from build123d import *

# Parameters (mm, degrees)
SKETCH1_W           = 20.5
SKETCH1_H           = 40.64
BOSS_EXTRUDE1_DEPTH = 39.5
CUT_EXTRUDE1_DEPTH  = 21.5
SKETCH3_W           = 55.64
SKETCH3_H           = 2.5
BOSS_EXTRUDE2_DEPTH = 20.5
SKETCH4_R           = 2.125
CUT_EXTRUDE2_DEPTH  = 33
SKETCH5_W           = 2.5
SKETCH5_H           = 1.601534114
CUT_EXTRUDE3_DEPTH  = 33
BOSS_EXTRUDE3_DEPTH = 1
SKETCH7_R           = 6.5
BOSS_EXTRUDE4_DEPTH = 1.5
SKETCH8_R           = 2.9
BOSS_EXTRUDE5_DEPTH = 1.25
SKETCH9_R           = 4.445
BOSS_EXTRUDE6_DEPTH = 3
SKETCH10_R          = 10.4
BOSS_EXTRUDE7_DEPTH = 2
SKETCH11_R          = 1.25
CUT_EXTRUDE4_DEPTH  = 7.75
SKETCH12_R          = 3.45
SKETCH12_R_2        = 2.85
BOSS_EXTRUDE8_DEPTH = 0.7
SKETCH13_R          = 0.4
CUT_EXTRUDE5_DEPTH  = 2
FILLET1_R           = 1.5
FILLET2_R           = 0.5
CUT_EXTRUDE6_START  = -7.75
CUT_EXTRUDE6_DEPTH  = 0.5
CUT_EXTRUDE7_DEPTH  = 0.5
SKETCH16_W          = 50.439593456
SKETCH16_H          = 8.25
CUT_EXTRUDE8_DEPTH  = 21.65
SKETCH17_R          = 8.5
BOSS_EXTRUDE9_DEPTH = 4


with BuildPart() as part:
    # Sketch1 → Boss-Extrude1 (new body)
    with BuildSketch(Plane(origin=(0, 0, 0), x_dir=(1, 0, 0), z_dir=(0, 1, 0))):
        with Locations((0, 20.32)):
            Rectangle(SKETCH1_W, SKETCH1_H)
    extrude(amount=BOSS_EXTRUDE1_DEPTH)

    # Sketch2 → Cut-Extrude1 (cut, through all)
    with BuildSketch(Plane(origin=(10.25, 0, 0), x_dir=(0, 0, -1), z_dir=(1, 0, 0))):
        Polygon((0, 39.5), (0, 36.35), (8, 39.5), align=None)
    extrude(amount=-CUT_EXTRUDE1_DEPTH, mode=Mode.SUBTRACT)

    # Sketch3 → Boss-Extrude2 (add)
    with BuildSketch(Plane(origin=(10.25, 0, 0), x_dir=(0, 0, -1), z_dir=(1, 0, 0))):
        with Locations((20.32, 30.75)):
            Rectangle(SKETCH3_W, SKETCH3_H)
    extrude(amount=-BOSS_EXTRUDE2_DEPTH)

    # Sketch4 → Cut-Extrude2 (cut, through all)
    with BuildSketch(Plane(origin=(0, 32, 0), x_dir=(1, 0, 0), z_dir=(0, 1, 0))):
        with Locations((-5, -4.18)):
            Circle(SKETCH4_R)
        with Locations((5, -4.18)):
            Circle(SKETCH4_R)
        with Locations((5, 44.82)):
            Circle(SKETCH4_R)
        with Locations((-5, 44.82)):
            Circle(SKETCH4_R)
    extrude(amount=-CUT_EXTRUDE2_DEPTH, mode=Mode.SUBTRACT)

    # Sketch5 → Cut-Extrude3 (cut, through all)
    with BuildSketch(Plane(origin=(0, 32, 0), x_dir=(1, 0, 0), z_dir=(0, 1, 0))):
        with Locations((5, -6.699232943)):
            Rectangle(SKETCH5_W, SKETCH5_H)
        with Locations((-5, -6.699232943)):
            Rectangle(SKETCH5_W, SKETCH5_H)
        with Locations((-5, 47.339232943)):
            Rectangle(SKETCH5_W, SKETCH5_H)
        with Locations((5, 47.339232943)):
            Rectangle(SKETCH5_W, SKETCH5_H)
    extrude(amount=-CUT_EXTRUDE3_DEPTH, mode=Mode.SUBTRACT)

    # Sketch6 → Boss-Extrude3 (add, symmetric)
    with BuildSketch(Plane(origin=(0, 0, 0), x_dir=(0, 0, -1), z_dir=(1, 0, 0))):
        Polygon((0, 32), (-5, 32), (0, 34.5), align=None)
        Polygon((40.64, 32), (45.64, 32), (40.64, 34.5), align=None)
    extrude(amount=BOSS_EXTRUDE3_DEPTH, both=True)

    # Sketch7 → Boss-Extrude4 (add)
    with BuildSketch(Plane(origin=(0, 39.5, 0), x_dir=(1, 0, 0), z_dir=(0, 1, 0))):
        with Locations((0, 30.14)):
            Circle(SKETCH7_R)
    extrude(amount=BOSS_EXTRUDE4_DEPTH)

    # Sketch8 → Boss-Extrude5 (add)
    with BuildSketch(Plane(origin=(0, 41, 0), x_dir=(1, 0, 0), z_dir=(0, 1, 0))):
        with Locations((0, 30.14)):
            Circle(SKETCH8_R)
    extrude(amount=BOSS_EXTRUDE5_DEPTH)

    # Sketch9 → Boss-Extrude6 (add)
    with BuildSketch(Plane(origin=(0, 42.25, 0), x_dir=(1, 0, 0), z_dir=(0, 1, 0))):
        with Locations((0, 30.14)):
            Circle(SKETCH9_R)
    extrude(amount=BOSS_EXTRUDE6_DEPTH)

    # Sketch10 → Boss-Extrude7 (add)
    with BuildSketch(Plane(origin=(0, 45.25, 0), x_dir=(1, 0, 0), z_dir=(0, 1, 0))):
        with Locations((0, 30.14)):
            Circle(SKETCH10_R)
    extrude(amount=BOSS_EXTRUDE7_DEPTH)

    # Sketch11 → Cut-Extrude4 (cut)
    with BuildSketch(Plane(origin=(0, 47.25, 0), x_dir=(1, 0, 0), z_dir=(0, 1, 0))):
        with Locations((0, 30.14)):
            Circle(SKETCH11_R)
    extrude(amount=-CUT_EXTRUDE4_DEPTH, mode=Mode.SUBTRACT)

    # Sketch12 → Boss-Extrude8 (add)
    with BuildSketch(Plane(origin=(0, 47.25, 0), x_dir=(1, 0, 0), z_dir=(0, 1, 0))):
        with Locations((0, 30.14)):
            Circle(SKETCH12_R)
        with Locations((0, 30.14)):
            Circle(SKETCH12_R_2, mode=Mode.SUBTRACT)
    extrude(amount=BOSS_EXTRUDE8_DEPTH)

    # Sketch13 → Cut-Extrude5 (cut)
    with BuildSketch(Plane(origin=(0, 47.25, 0), x_dir=(1, 0, 0), z_dir=(0, 1, 0))):
        with Locations((0, 37.265)):
            Circle(SKETCH13_R)
        with Locations((3.5, 37.265)):
            Circle(SKETCH13_R)
        with Locations((-3.5, 37.265)):
            Circle(SKETCH13_R)
        with Locations((7.125, 26.64)):
            Circle(SKETCH13_R)
        with Locations((7.125, 30.14)):
            Circle(SKETCH13_R)
        with Locations((7.125, 33.64)):
            Circle(SKETCH13_R)
        with Locations((-3.5, 23.015)):
            Circle(SKETCH13_R)
        with Locations((0, 23.015)):
            Circle(SKETCH13_R)
        with Locations((3.5, 23.015)):
            Circle(SKETCH13_R)
        with Locations((-7.125, 33.64)):
            Circle(SKETCH13_R)
        with Locations((-7.125, 30.14)):
            Circle(SKETCH13_R)
        with Locations((-7.125, 26.64)):
            Circle(SKETCH13_R)
    extrude(amount=-CUT_EXTRUDE5_DEPTH, mode=Mode.SUBTRACT)

    # Fillet1
    fillet1_edges = [part.edges().sort_by_distance(p)[0] for p in [
        (10.25, 34.175, 0),
        (-10.25, 34.175, 0),
        (-10.25, 14.75, -40.64),
        (10.25, 14.75, -40.64),
        (10.25, 14.75, 0),
        (-10.25, 14.75, 0),
        (-10.25, 35.75, -40.64),
        (10.25, 35.75, -40.64),
    ]]
    fillet(fillet1_edges, radius=FILLET1_R)

    # Fillet2
    fillet2_edges = [part.edges().sort_by_distance(p)[0] for p in [
        (-3.75, 30.75, -48.14),
        (-6.25, 30.75, -48.14),
        (3.75, 30.75, -48.14),
        (6.25, 30.75, -48.14),
        (10.25, 30.75, 7.5),
        (-10.25, 30.75, 7.5),
        (-10.25, 30.75, -48.14),
        (-3.75, 30.75, 7.5),
        (-6.25, 30.75, 7.5),
        (3.75, 30.75, 7.5),
        (6.25, 30.75, 7.5),
    ]]
    fillet(fillet2_edges, radius=FILLET2_R)

    # Sketch14 → Cut-Extrude6 (cut)
    with BuildSketch(Plane.XZ.offset(CUT_EXTRUDE6_START)):
        with BuildLine():
            Line((-8.75, -40.64), (8.75, -40.64))
            ThreePointArc((8.75, -40.64), (9.810660172, -40.200660172), (10.25, -39.14))
            Line((10.25, -39.14), (10.25, -1.5))
            ThreePointArc((10.25, -1.5), (9.810660172, -0.439339828), (8.75, 0))
            Line((8.75, 0), (-8.75, 0))
            ThreePointArc((-8.75, 0), (-9.810660172, -0.439339828), (-10.25, -1.5))
            Line((-10.25, -1.5), (-10.25, -39.14))
            ThreePointArc((-10.25, -39.14), (-9.810660172, -40.200660172), (-8.75, -40.64))
        make_face()
        with BuildLine():
            Line((8.75, -0.25), (-8.75, -0.25))
            ThreePointArc((-8.75, -0.25), (-9.633883476, -0.616116524), (-10, -1.5))
            Line((-10, -1.5), (-10, -39.14))
            ThreePointArc((-10, -39.14), (-9.633883476, -40.023883476), (-8.75, -40.39))
            Line((-8.75, -40.39), (8.75, -40.39))
            ThreePointArc((8.75, -40.39), (9.633883476, -40.023883476), (10, -39.14))
            Line((10, -39.14), (10, -1.5))
            ThreePointArc((10, -1.5), (9.633883476, -0.616116524), (8.75, -0.25))
        make_face(mode=Mode.SUBTRACT)
    extrude(amount=-CUT_EXTRUDE6_DEPTH, mode=Mode.SUBTRACT)

    # Sketch15 → Cut-Extrude7 (cut)
    with BuildSketch(Plane.XZ.offset(-29.5)):
        with BuildLine():
            Line((-8.75, -40.64), (8.75, -40.64))
            ThreePointArc((8.75, -40.64), (9.810660172, -40.200660172), (10.25, -39.14))
            Line((10.25, -39.14), (10.25, -1.5))
            ThreePointArc((10.25, -1.5), (9.810660172, -0.439339828), (8.75, 0))
            Line((8.75, 0), (-8.75, 0))
            ThreePointArc((-8.75, 0), (-9.810660172, -0.439339828), (-10.25, -1.5))
            Line((-10.25, -1.5), (-10.25, -39.14))
            ThreePointArc((-10.25, -39.14), (-9.810660172, -40.200660172), (-8.75, -40.64))
        make_face()
        with BuildLine():
            Line((10, -39.14), (10, -1.5))
            ThreePointArc((10, -1.5), (9.633883476, -0.616116524), (8.75, -0.25))
            Line((8.75, -0.25), (-8.75, -0.25))
            ThreePointArc((-8.75, -0.25), (-9.633883476, -0.616116524), (-10, -1.5))
            Line((-10, -1.5), (-10, -39.14))
            ThreePointArc((-10, -39.14), (-9.633883476, -40.023883476), (-8.75, -40.39))
            Line((-8.75, -40.39), (8.75, -40.39))
            ThreePointArc((8.75, -40.39), (9.633883476, -40.023883476), (10, -39.14))
        make_face(mode=Mode.SUBTRACT)
    extrude(amount=CUT_EXTRUDE7_DEPTH, mode=Mode.SUBTRACT)

    # Sketch16 → Cut-Extrude8 (cut, through all)
    with BuildSketch(Plane(origin=(10.25, 0, 0), x_dir=(0, 0, -1), z_dir=(1, 0, 0))):
        with Locations((25.219796728, 4.125)):
            Rectangle(SKETCH16_W, SKETCH16_H)
    extrude(amount=-CUT_EXTRUDE8_DEPTH, mode=Mode.SUBTRACT)

    # Sketch17 → Boss-Extrude9 (add)
    with BuildSketch(Plane.XZ.offset(-8.25)):
        with Locations((0, -10.5)):
            Circle(SKETCH17_R)
    extrude(amount=BOSS_EXTRUDE9_DEPTH)


solid = part.part
Design review of the part built by this model. Coordinates are the model's own, in mm. A direction names the side the tool comes from. Coordinates: 2 decimals unless noted, no trailing zeros. Order: outer loops, then holes, each group sorted by start corner. A loop starts at its lowest first (then second) coordinate and runs counter-clockwise, first axis right, second up.
Item 1: For pin 1 Ø10 at (x, y) = (2.5, 20) entering from -Z; pin 2 Ø10 at (y, z) = (31, -24.5) entering from -X; pin 3 Ø1.2 at (y, z) = (31, 6) entering from +X; pin 4 Ø4 at (x, z) = (-5, 4.18) entering from -Y, all flat-tipped, find the tip position at first contact; note any pin that passes through.
Item 2: For faces 1 (the flat face through (0, 42.25, -27)), 2 (the flat face through (-1, 33, 1)), 3 (the cylindrical face through (9.8, 35.8, -40.21)), 4 (the flat face through (0, 39.5, -30)), list the 3-axis set-ups (+Z, -Z, +X, -X, +Y, -Y) from which the entire face can be reached by the end or side of a thin tool; tool diameter is ignored.
Item 3: Take a section at C-C, the plane z = -21. Write out the cut boundary in (x, y), then the cut area to 3 significant figures.
Item 4: Take a section at B-B, the plane y = 21. Write out the cut boundary in (x, z), then the cut area to 3 significant figures.
Item 5: Take a section at D-D, the plane y = 43.5. Write out the cut boundary in (x, z) (3 decimals).
Item 6: The part is to be moulded in two halves that separate along Z. For faces 5 (the flat face through (0, 36, -40.64)), 6 (the flat face through (0.14, 37.9, -3.94)), 7 (the cylindrical face through (-0.62, 47.6, -27.36)), say which applies: pulls with the +Z half, pulls with the -Z half, needs draft (parallel to the pull), parting line crosses it, or undercut.
Item 7: For line 1 (Y direction, x = 6, z = -22); line 2 (Z direction, x = -3.5, y = 46.3) (3 decimals); line 3 (X direction, y = 46, z = -30), list the stretches that pass through material, from the lowest coordinate up.
Item 8: Take a section at A-A, the plane z = -44.82. Write out the cut boundary in (x, y) (3 decimals), then the cut area to 3 significant figures.
The answers:
1. pin 1: stops at z = -40.64
1. pin 2: stops at x = -10.25
1. pin 3: stops at x = 10.25
1. pin 4: passes through
2. face 1: none
2. face 2: +Z, -X, +Y
2. face 3: -Z, +X, +Y
2. face 4: +Y
3. outline: (-10.25, 8.25) - (10.25, 8.25) - (10.25, 29) - (10, 29) - (10, 29.5) - (10.25, 29.5) - (10.25, 39.5) - (-10.25, 39.5) - (-10.25, 29.5) - (-10, 29.5) - (-10, 29) - (-10.25, 29) - close; (-4.96, 45.25) - (4.96, 45.25) - (4.96, 47.25) - (-4.96, 47.25) - close
3. area: 660 mm2
4. outline: (-10.25, -39.14) arc R1.5 ccw to (-8.75, -40.64) - (8.75, -40.64) arc R1.5 ccw to (10.25, -39.14) - (10.25, -1.5) arc R1.5 ccw to (8.75, 0) - (-8.75, 0) arc R1.5 ccw to (-10.25, -1.5) - close
4. area: 831 mm2
5. outline: circle Ø8.89 at (0, -30.14); hole circle Ø2.5 at (0, -30.14)
6. face 5: pulls with the -Z half
6. face 6: pulls with the +Z half
6. face 7: undercut
7. line 1: y = 8.25 to 39.5, 45.25 to 47.25
7. line 2: z = -39.933 to -37.665, -36.865 to -23.415, -22.615 to -20.347
7. line 3: x = -10.4 to -7.5, -6.75 to -1.24, 1.24 to 6.75, 7.5 to 10.4
8. outline: (-10.25, 29.5) - (-7.125, 29.5) - (-7.125, 32) - (-10.25, 32) - close; (-2.875, 29.5) - (2.875, 29.5) - (2.875, 32) - (1, 32) - (1, 32.41) - (-1, 32.41) - (-1, 32) - (-2.875, 32) - close; (7.125, 29.5) - (10.25, 29.5) - (10.25, 32) - (7.125, 32) - close
8. area: 30.8 mm2
